For this review, take the finished solid that the model builds, in its own axes (mm). A direction names the side the tool comes from. Coordinates: 2 decimals unless noted, no trailing zeros. Write each loop counter-clockwise with the first axis right and the second up, starting at its lowest first coordinate (ties: lowest second). Pieces come first, ordered by that corner, then holes. Notation, with made-up numbers: M 12,8.5 L 17,8.5 A26 ccw 17,40.5 Z; hole C -25.5,26.25 d7. An arc over 180 degrees is marked long. One line per question, with ' | ' between items.
from build123d import *

# Parameters (mm, degrees)
F1_DEPTH       = 60
F2_R           = 1.49999
F4_D           = 4.2
F4_CBORE_D     = 9.75
F4_CBORE_DEPTH = 4


# Not quite as in the source:
# - a fillet or chamfer is up to 0.001 mm smaller than in the source, because OpenCascade refuses the exact size
# - a feature names something its author has since deleted; it is built from what else it names


with BuildPart() as f1:
    # F0 (on Right) → F1 (new body)
    with BuildSketch(Plane.YZ):
        Polygon((10, 1.9290046394), (4, 1.9290046394), (4, -38.0709953606), (-20, -38.0709953606), (-20, -41.0709953606), (10, -41.0709953606), (10, -34.6), (11.5, -33.1), (11.5, -26.9), (10, -25.4), (10, -14.6), (11.5, -13.1), (11.5, -6.9), (10, -5.4), align=None)
    extrude(amount=-F1_DEPTH)

    # F2 (radius 1.5 in the source; OpenCascade refuses exactly that, so slightly less here)
    f2_edges = [f1.edges().sort_by_distance(p)[0] for p in [
        (0, 4, -18.070995),
        (-60, 4, -18.070995),
        (0, -8, -38.070995),
        (-30, -20, -38.070995),
        (-60, -8, -38.070995),
        (-30, 4, -38.070995),
        (-30, -20, -41.070995),
        (0, -5, -41.070995),
        (-60, -5, -41.070995),
        (-30, 4, 1.929005),
    ]]
    fillet(f2_edges, radius=F2_R)

    # F4 (through all)
    with Locations(Plane.XZ.offset(-4)):
        with Locations((-30, -9.9999953606), (-30, -29.9999953606)):
            CounterBoreHole(F4_D / 2, F4_CBORE_D / 2, F4_CBORE_DEPTH)


solid = f1.part
1) We need section A-A on x = -30. State how many separate pieces and enclosed holes the cut face has, then the cut area to 3 significant figures.
Responses:
separate pieces: 3 | enclosed holes: 0 | area: 245 mm^2
2) Insertion check: pin 1 Ø3.5 at (x, z) = (-31, 0) entering from +Y; pin 2 Ø1 at (x, z) = (-35.5, -12) entering from -Y; pin 3 Ø6 at (x, z) = (-30, -10) entering from -Y; pin 4 Ø12 at (x, z) = (-25, -19) entering from +Y. Each pin has a flat end and moves straight along its axis. Give the tip position at first contact, or say it passes through.
Responses:
pin 1: y = 10 | pin 2: y = 4 | pin 3: y = 8 | pin 4: y = 11.5
3) Machinability: for faces 1 (the flat face through (-30, 10, -38)), 2 (the flat face through (-29, 8, -12.1)), 3 (the cylindrical face through (-59.55, 4.43, -17.59)), 4 (the flat face through (-29.6, 10.8, -26.2)), which of the approach directions +Z, -Z, +X, -X, +Y, -Y give a long, thin tool a straight path to every point of the face, cutting with its end or side? Answer none if there is none.
Responses:
face 1: -Z, +X, -X, +Y | face 2: -Y | face 3: +Z, -X, -Y | face 4: +X, -X, +Y
4) We need section C-C on z = -17.5. State the section outline as (x, y) points, then the cut area to 3 significant figures.
Responses:
outline: M -60,5.5 A1.5 ccw -58.5,4 L -1.5,4 A1.5 ccw 0,5.5 L 0,10 L -60,10 Z | area: 359 mm^2
5) To check wall thickness, follow line 1 along Z through (x, y) = (-30, 6) (3 decimals); line 2 along Z through (x, y) = (-30, 9); line 3 along Z through (x, y) = (-30, 10.8). State the ranges of each line that lie inside material, in increasing order. Write a range as [from, to].
Responses:
line 1: [-41.071, -34.875], [-25.125, -14.875], [-5.125, 1.929] | line 2: [-41.07, -32.1], [-27.9, -12.1], [-7.9, 1.93] | line 3: [-33.8, -32.1], [-27.9, -26.2], [-13.8, -12.1], [-7.9, -6.2]
6) The part is to be moulded in two halves that separate along X. For faces 5 (the flat face through (-30, -4, -41.071)), 6 (the cylindrical face through (-34.87, 5.97, -9.79)), 7 (the cylindrical face through (-0.45, -8.91, -38.5)), say which applies: +X half, -X half, draft (parallel to the pull), parting line (faces both ways), or undercut.
Responses:
face 5: draft | face 6: undercut | face 7: +X half
